```python
from build123d import *

# Parameters (mm, degrees)
BOSS_EXTRUDE1_DEPTH     = 25
SKETCH2_R               = 2
CUT_EXTRUDE1_DEPTH      = 155.056807704
SKETCH4_R               = 2
CUT_EXTRUDE2_DEPTH      = 155.056807704
LPATTERN1_COUNT         = 5
LPATTERN1_PITCH         = 56.5
MIRROR2_COPY_1_SKETCH_R = 2
MIRROR2_COPY_1_DEPTH    = 155.056807704
MIRROR2_COPY_2_SKETCH_R = 2
MIRROR2_COPY_2_DEPTH    = 155.056807704
MIRROR2_COPY_3_SKETCH_R = 2
MIRROR2_COPY_3_DEPTH    = 155.056807704
MIRROR2_COPY_4_SKETCH_R = 2
MIRROR2_COPY_4_DEPTH    = 155.056807704
BOSS_EXTRUDE2_DEPTH     = 235


with BuildPart() as part:
    # Sketch1 → Boss-Extrude1 (new body)
    with BuildSketch(Plane.XY):
        with BuildLine():
            Line((-32.5, -116), (-32.5, 116))
            ThreePointArc((-32.5, 116), (0, 148.5), (32.5, 116))
            Line((32.5, 116), (32.5, -116))
            ThreePointArc((32.5, -116), (0, -148.5), (-32.5, -116))
        make_face()
        with BuildLine():
            Line((-25.5, -116), (-25.5, 116))
            ThreePointArc((-25.5, 116), (0, 141.5), (25.5, 116))
            Line((25.5, 116), (25.5, -116))
            ThreePointArc((25.5, -116), (0, -141.5), (-25.5, -116))
        make_face(mode=Mode.SUBTRACT)
    extrude(amount=BOSS_EXTRUDE1_DEPTH)

    # Sketch2 → Cut-Extrude1 (cut, through all)
    with BuildSketch(Plane.XY.offset(25)):
        with Locations((-5, 144)):
            Circle(SKETCH2_R)
        with Locations((5, 144)):
            Circle(SKETCH2_R)
    cut_extrude1 = extrude(amount=-CUT_EXTRUDE1_DEPTH, mode=Mode.SUBTRACT)

    # Mirror1: Cut-Extrude1 across plane
    add(cut_extrude1.mirror(Plane.ZX), mode=Mode.SUBTRACT)

    # Sketch4 → Cut-Extrude2 (cut, through all)
    with BuildSketch(Plane.XY.offset(25)):
        with Locations((28.5, 116)):
            Circle(SKETCH4_R)
    cut_extrude2 = extrude(amount=-CUT_EXTRUDE2_DEPTH, mode=Mode.SUBTRACT)

    # LPattern1: Cut-Extrude2 ×5
    with Locations(*[(0, -i * LPATTERN1_PITCH, 0) for i in range(1, LPATTERN1_COUNT)]):
        add(cut_extrude2, mode=Mode.SUBTRACT)

    # Mirror2: Cut-Extrude2 across plane
    add(cut_extrude2.mirror(Plane(origin=(0, 0, 0), x_dir=(0, 0, 1), z_dir=(1, 0, 0))), mode=Mode.SUBTRACT)

    # Mirror2 copy 1 sketch → Mirror2 copy 1 (cut, through all)
    with BuildSketch(Plane(origin=(0, -56.5, 25), x_dir=(-1, 0, 0), z_dir=(0, 0, 1))):
        with Locations((28.5, -116)):
            Circle(MIRROR2_COPY_1_SKETCH_R)
    extrude(amount=-MIRROR2_COPY_1_DEPTH, mode=Mode.SUBTRACT)

    # Mirror2 copy 2 sketch → Mirror2 copy 2 (cut, through all)
    with BuildSketch(Plane(origin=(0, -113, 25), x_dir=(-1, 0, 0), z_dir=(0, 0, 1))):
        with Locations((28.5, -116)):
            Circle(MIRROR2_COPY_2_SKETCH_R)
    extrude(amount=-MIRROR2_COPY_2_DEPTH, mode=Mode.SUBTRACT)

    # Mirror2 copy 3 sketch → Mirror2 copy 3 (cut, through all)
    with BuildSketch(Plane(origin=(0, -169.5, 25), x_dir=(-1, 0, 0), z_dir=(0, 0, 1))):
        with Locations((28.5, -116)):
            Circle(MIRROR2_COPY_3_SKETCH_R)
    extrude(amount=-MIRROR2_COPY_3_DEPTH, mode=Mode.SUBTRACT)

    # Mirror2 copy 4 sketch → Mirror2 copy 4 (cut, through all)
    with BuildSketch(Plane(origin=(0, -226, 25), x_dir=(-1, 0, 0), z_dir=(0, 0, 1))):
        with Locations((28.5, -116)):
            Circle(MIRROR2_COPY_4_SKETCH_R)
    extrude(amount=-MIRROR2_COPY_4_DEPTH, mode=Mode.SUBTRACT)

    # Sketch5 → Boss-Extrude2 (add)
    with BuildSketch(Plane(origin=(32.5, 116, 0), x_dir=(1, 0, 0), z_dir=(0, 1, 0))):
        with BuildLine():
            Line((0, 0), (7, 0))
            ThreePointArc((7, 0), (19.5, -12.5), (7, -25))
            Line((7, -25), (7, -23))
            ThreePointArc((7, -23), (17.5, -12.5), (7, -2))
            Line((7, -2), (0, -2))
            Line((0, -2), (0, 0))
        make_face()
    extrude(amount=-BOSS_EXTRUDE2_DEPTH)


solid = part.part
```
The listing builds one solid part. Answer for the finished solid, in the listing's coordinates (mm). A direction names the side the tool comes from. Give positions to 0.01 mm unless a question says otherwise; leave off trailing zeros. Loops run counter-clockwise (first coordinate to the right, second up) from the corner with the lowest first, then second, coordinate; pieces in that order, holes last. Notation, with made-up numbers: M 16.5,87.5 L 72.5,87.5 A10 cw 72.5,98.5 Z; hole C -25.75,51 d6. An arc over 180 degrees is marked long. One line per item, written item: value.
1. For faces 5 (the face through (-0.561, 141.494, 12.325)), 6 (the face through (27, 23, 25)), 7 (the face through (50, 0.1, 12.7)), 8 (the face through (32.5, 2, 13)), 9 (the face through (50, 116, 9)), determine the directions among +Z, -Z, +X, -X, +Y, -Y from which every point of the face is accessible in a straight line to the end or side of a thin tool.
Found:
face 5: +Z, -Z
face 6: +Z, +X, -X, +Y, -Y
face 7: +Y, -Y
face 8: +Z, +Y, -Y
face 9: +Z, -Z, +X, +Y
2. Section C-C on x = 42.5 is taken. Determine the outline of the cut face in (y, z).
Found:
outline: M -119,0.37 L 116,0.37 L 116,2.44 L -119,2.44 Z; M -119,22.56 L 116,22.56 L 116,24.63 L -119,24.63 Z
3. Each of these flat-tipped pins is pushed along its axis until it touches: P1, Ø1.5, axis at x = -1, z = 4.5, coming from the -Y side; P2, Ø5, axis at x = -23, z = 10, coming from the +Y side; P3, Ø4, axis at y = -62, z = 20, coming from the +X side (3 decimals). Where does it stop, or does it pass through?
Found:
P1: y = -148.5
P2: y = 141.22
P3: x = 50.725
4. Find the intervals of material crossed by probe 1 along X at (y, z) = (108, 14.25); probe 2 along Y at (x, z) = (-29, 16); probe 3 along Y at (x, z) = (-28.5, 15.5), in increasing order.
Found:
probe 1: -32.5 to -25.5, 25.5 to 32.5, 49.85 to 51.88
probe 2: -130.67 to -111.94, -108.06 to -55.44, -51.56 to 1.06, 4.94 to 57.56, 61.44 to 114.06, 117.94 to 130.67
probe 3: -131.62 to -112, -108 to -55.5, -51.5 to 1, 5 to 57.5, 61.5 to 114, 118 to 131.62
5. Section A-A on y = 99 is taken. Determine the outline of the cut face in (x, z), plus the area to 3 significant figures.
Found:
outline: M -32.5,0 L -25.5,0 L -25.5,25 L -32.5,25 Z; M 25.5,0 L 39.5,0 A12.5 ccw 39.5,25 L 39.5,23 A10.5 cw 39.5,2 L 32.5,2 L 32.5,25 L 25.5,25 Z
area: 436 mm^2
6. For a pull along X with two mould halves and no side action, classify faces 1 (the face through (50, -119, 9)), 2 (the face through (-25.5, -2, 12)), 3 (the face through (-0.715, 148.492, 12.325)), 4 (the face through (51.997, 0.145, 12.225)) as pulls with the +X half, pulls with the -X half, needs draft (parallel to the pull), parting line crosses it, or undercut.
Found:
face 1: needs draft
face 2: undercut
face 3: parting line crosses it
face 4: pulls with the +X half
7. Section B-B on z = 10.75 is taken. State how many separate pieces and enclosed holes the cut face has, plus the area to 3 significant figures.
Found:
separate pieces: 2
enclosed holes: 15
area: 4,820 mm^2
